Check sheet for the modelled part. Datum: model origin and axes. Units: mm. A direction names the side the tool comes from. Round coordinates to 2 decimals unless told otherwise and drop trailing zeros. Order: outer loops, then holes, each group sorted by start corner. A loop starts at its lowest first (then second) coordinate and runs counter-clockwise, first axis right, second up.
```python
from build123d import *

# Parameters (mm, degrees)
BASE_FLANGE1_DEPTH = 44.45
SKETCH6_W          = 31.75
SKETCH6_H          = 3.429
CUT_EXTRUDE1_DEPTH = 287.781062931
SKETCH7_W          = 31.75
SKETCH7_H          = 3.429
CUT_EXTRUDE2_DEPTH = 275.16810415


# Sheet-metal steps are written as plain solids
with BuildPart() as part:
    # Sketch1 → Base-Flange1 (new body)
    with BuildSketch(Plane(origin=(0, 0, 0), x_dir=(1, 0, 0), z_dir=(0, 1, 0))):
        with BuildLine():
            Line((0, 0), (196.990405775, 0))
            ThreePointArc((196.990405775, 0), (197.677601549, 0.075260177), (198.332218756, 0.297472776))
            Line((198.332218756, 0.297472776), (279.4, 38.1))
            Line((279.4, 38.1), (280.741812981, 35.222472776))
            Line((280.741812981, 35.222472776), (199.674031737, -2.580054448))
            ThreePointArc((199.674031737, -2.580054448), (198.364797323, -3.024479645), (196.990405775, -3.175))
            Line((196.990405775, -3.175), (0, -3.175))
            Line((0, -3.175), (0, 0))
        make_face()
    extrude(amount=BASE_FLANGE1_DEPTH)

    # Sketch6 → Cut-Extrude1 (cut, through all)
    with BuildSketch(Plane(origin=(0, 0, 0), x_dir=(-1, 0, 0), z_dir=(0, 0, -1))):
        with Locations((-139.7, 7.9375)):
            Rectangle(SKETCH6_W, SKETCH6_H)
        with Locations((-63.5, 36.5125)):
            Rectangle(SKETCH6_W, SKETCH6_H)
        with Locations((-139.7, 36.5125)):
            Rectangle(SKETCH6_W, SKETCH6_H)
        with Locations((-63.5, 7.9375)):
            Rectangle(SKETCH6_W, SKETCH6_H)
    extrude(amount=-CUT_EXTRUDE1_DEPTH, mode=Mode.SUBTRACT)

    # Sketch7 → Cut-Extrude2 (cut, through all)
    with BuildSketch(Plane(origin=(35.309424285, 0, 75.721304739), x_dir=(-0.9063077870366493, 0, 0.42261826174070083), z_dir=(-0.4226182617407009, 0, -0.9063077870366494))):
        with Locations((-231.22415147, 36.5125)):
            Rectangle(SKETCH7_W, SKETCH7_H)
        with Locations((-231.22415147, 7.9375)):
            Rectangle(SKETCH7_W, SKETCH7_H)
    extrude(amount=-CUT_EXTRUDE2_DEPTH, mode=Mode.SUBTRACT)


solid = part.part
```
Item 1: Release check for a two-part mould opening along Y. For faces 3 (the flat face through (240.78, 21.91, -16.59)), 4 (the flat face through (151, 44.45, 1)), 5 (the flat face through (151, 0, 1)), 6 (the flat face through (246, 6.223, -21)) record: released by +Y, released by -Y, zero draft, split by the parting line, or undercut.
Answer:
face 3: zero draft
face 4: released by +Y
face 5: released by -Y
face 6: undercut
Item 2: Access from +Z, -Z, +X, -X, +Y, -Y to the whole of each face (thin tool, end or side, straight path). Record for faces 1 (the flat face through (100, 22, 3.175)), 2 (the flat face through (97, 22, 0)).
Answer:
face 1: +Z, +X, -X, +Y, -Y
face 2: -Z, -X, +Y, -Y
Item 3: Sectioned sample at B-B (y = 19). Record the cut outline in (x, z) (3 decimals).
Answer:
outline: (0, 0) - (196.99, 0) arc R3.175 cw to (198.332, -0.297) - (279.4, -38.1) - (280.742, -35.222) - (199.674, 2.58) arc R6.35 ccw to (196.99, 3.175) - (0, 3.175) - close
Item 4: Go/stop test with flat-tipped pins: P1, Ø1, axis at y = 36, z = 1.5, coming from the -X side; P2, Ø4, axis at y = 14.5, z = -6, coming from the -X side; P3, Ø10, axis at y = 22, z = -30.5, coming from the -X side; P4, Ø2, axis at y = 33, z = -3.5, coming from the +X side. Record where each tip stops, or that it passes through.
Answer:
P1: stops at x = 0
P2: stops at x = 206.27
P3: stops at x = 252.38
P4: stops at x = 214.86
Item 5: Sectioned sample at D-D (x = 242). Record the cut outline in (y, z), and give its area (3 significant figures).
Answer:
outline: (0, -20.66) - (6.22, -20.66) - (6.22, -17.16) - (0, -17.16) - close; (9.65, -20.66) - (34.8, -20.66) - (34.8, -17.16) - (9.65, -17.16) - close; (38.23, -20.66) - (44.45, -20.66) - (44.45, -17.16) - (38.23, -17.16) - close
area: 132 mm2
Item 6: Scan lines: line 1 along Z through (x, y) = (54.5, 28.5) (3 decimals); line 2 along X through (y, z) = (29, -1.5); line 3 along X through (y, z) = (29, -15). Record each from-to range of solid material in increasing order.
Answer:
line 1: z = 0 to 3.175
line 2: x = 200.91 to 208.42
line 3: x = 229.86 to 237.37
Item 7: Sectioned sample at A-A (x = 73). Record the cut outline in (y, z) (3 decimals).
Answer:
outline: (0, 0) - (6.223, 0) - (6.223, 3.175) - (0, 3.175) - close; (9.652, 0) - (34.798, 0) - (34.798, 3.175) - (9.652, 3.175) - close; (38.227, 0) - (44.45, 0) - (44.45, 3.175) - (38.227, 3.175) - close
Item 8: Sectioned sample at C-C (x = 174). Record the cut outline in (y, z) (3 decimals).
Answer:
outline: (0, 0) - (44.45, 0) - (44.45, 3.175) - (0, 3.175) - close
